Design review of the part built by this model. Coordinates are the model's own, in mm. A direction names the side the tool comes from. Round coordinates to 2 decimals unless told otherwise and drop trailing zeros. Order: outer loops, then holes, each group sorted by start corner. A loop starts at its lowest first (then second) coordinate and runs counter-clockwise, first axis right, second up. Notation, with made-up numbers: (-11.5, 24) - (22.5, 24) arc R28 cw to (22.5, 57) - close; hole circle Ø3 at (1.25, 31). An arc over 180 degrees is marked (long way). Answer as a JSON object with one key per item and string values. Group by question number.
from build123d import *

# Parameters (mm, degrees)
BOSS_EXTRUDE1_DEPTH = 30
SKETCH2_R           = 30
SKETCH2_R_2         = 12.5
CUT_EXTRUDE1_DEPTH  = 146.129146151
BOSS_EXTRUDE2_START = 90
SKETCH3_R           = 12.5
BOSS_EXTRUDE2_DEPTH = 90
BOSS_EXTRUDE3_START = -140
SKETCH3_2_R         = 12.5
BOSS_EXTRUDE3_DEPTH = 90
SKETCH4_W           = 30
SKETCH4_H           = 25
BOSS_EXTRUDE4_DEPTH = 5
SKETCH8_W           = 30
SKETCH8_H           = 5
BOSS_EXTRUDE7_DEPTH = 25
SKETCH9_R           = 4
CUT_EXTRUDE2_DEPTH  = 242.111266906


with BuildPart() as part:
    # Sketch1 → Boss-Extrude1 (new body)
    with BuildSketch(Plane.XY):
        Polygon((20.439052972, 3.783569778), (18.715311494, 3.783569778), (17.077445439, 8.283569778), (15.793733726, 8.283569778), (14.155867672, 3.783569778), (12.432126194, 3.783569778), (10.794260139, 8.283569778), (9.510548426, 8.283569778), (7.872682372, 3.783569778), (6.148940894, 3.783569778), (4.511074839, 8.283569778), (3.227363126, 8.283569778), (1.589497072, 3.783569778), (-0.134244406, 3.783569778), (-1.772110461, 8.283569778), (-3.055822174, 8.283569778), (-4.693688228, 3.783569778), (-6.417429706, 3.783569778), (-8.055295761, 8.283569778), (-9.339007474, 8.283569778), (-10.976873528, 3.783569778), (-12.700615006, 3.783569778), (-14.338481061, 8.283569778), (-15.622192774, 8.283569778), (-17.260058828, 3.783569778), (-18.983800306, 3.783569778), (-20.621666361, 8.283569778), (-21.905378074, 8.283569778), (-23.543244128, 3.783569778), (-25.266985606, 3.783569778), (-26.904851661, 8.283569778), (-28.188563374, 8.283569778), (-29.826429428, 3.783569778), (-31.550170906, 3.783569778), (-33.188036961, 8.283569778), (-34.471748674, 8.283569778), (-36.109614728, 3.783569778), (-37.833356206, 3.783569778), (-39.471222261, 8.283569778), (-40.754933974, 8.283569778), (-42.392800028, 3.783569778), (-44.116541506, 3.783569778), (-45.754407561, 8.283569778), (-47.038119274, 8.283569778), (-48.675985328, 3.783569778), (-50.399726806, 3.783569778), (-52.037592861, 8.283569778), (-53.321304574, 8.283569778), (-54.959170628, 3.783569778), (-56.682912106, 3.783569778), (-58.320778161, 8.283569778), (-59.604489874, 8.283569778), (-61.242355928, 3.783569778), (-62.966097406, 3.783569778), (-64.603963461, 8.283569778), (-65.887675174, 8.283569778), (-67.525541228, 3.783569778), (-69.249282706, 3.783569778), (-70.887148761, 8.283569778), (-72.170860474, 8.283569778), (-73.808726528, 3.783569778), (-75.532468006, 3.783569778), (-77.170334061, 8.283569778), (-78.454045774, 8.283569778), (-80.091911828, 3.783569778), (-81.815653306, 3.783569778), (-83.453519361, 8.283569778), (-84.737231074, 8.283569778), (-86.375097128, 3.783569778), (-88.098838606, 3.783569778), (-89.736704661, 8.283569778), (-91.020416374, 8.283569778), (-92.658282428, 3.783569778), (-94.382023906, 3.783569778), (-96.019889961, 8.283569778), (-97.303601674, 8.283569778), (-98.941467728, 3.783569778), (-100.665209206, 3.783569778), (-102.303075261, 8.283569778), (-103.586786974, 8.283569778), (-105.224653028, 3.783569778), (-106.948394506, 3.783569778), (-108.586260561, 8.283569778), (-109.869972274, 8.283569778), (-111.507838328, 3.783569778), (-113.231579806, 3.783569778), (-114.869445861, 8.283569778), (-116.153157574, 8.283569778), (-117.791023628, 3.783569778), (-118.652894367, 3.783569778), (-118.652894367, -23.716430222), (21.347105633, -23.716430222), (21.347105633, 6.278423959), align=None)
    extrude(amount=BOSS_EXTRUDE1_DEPTH)

    # Sketch2 → Cut-Extrude1 (cut, through all)
    with BuildSketch(Plane.ZY.offset(118.652894367)):
        with Locations((15, -4.216430222)):
            Circle(SKETCH2_R)
        with Locations(Location((15, -4.216430222, 0), (0, 0, 39.7918195))):
            Circle(SKETCH2_R_2, mode=Mode.SUBTRACT)
    extrude(amount=-CUT_EXTRUDE1_DEPTH, mode=Mode.SUBTRACT)

    # Sketch3 → Boss-Extrude2 (add)
    with BuildSketch(Plane.ZY.offset(118.652894367).offset(BOSS_EXTRUDE2_START)):
        with Locations((15, -4.216430222)):
            Circle(SKETCH3_R)
    extrude(amount=-BOSS_EXTRUDE2_DEPTH)

    # Sketch3_2 → Boss-Extrude3 (add)
    with BuildSketch(Plane.ZY.offset(118.652894367).offset(BOSS_EXTRUDE3_START)):
        with Locations((15, -4.216430222)):
            Circle(SKETCH3_2_R)
    extrude(amount=-BOSS_EXTRUDE3_DEPTH)

    # Sketch4 → Boss-Extrude4 (add)
    with BuildSketch(Plane.ZY.offset(208.652894367)):
        with Locations((15, -4.216430222)):
            Rectangle(SKETCH4_W, SKETCH4_H)
    boss_extrude4 = extrude(amount=BOSS_EXTRUDE4_DEPTH)

    # Sketch8 → Boss-Extrude7 (add)
    with BuildSketch(Plane(origin=(0, 8.283569778, 0), x_dir=(1, 0, 0), z_dir=(0, 1, 0))):
        with Locations((-223.652894367, -2.5)):
            Rectangle(SKETCH8_W, SKETCH8_H)
        with Locations((-223.652894367, -27.5)):
            Rectangle(SKETCH8_W, SKETCH8_H)
    boss_extrude7 = extrude(amount=-BOSS_EXTRUDE7_DEPTH)

    # Sketch9 → Cut-Extrude2 (cut, through all)
    with BuildSketch(Plane.XY.offset(30)):
        with Locations((-229.652894367, -4.216430222)):
            Circle(SKETCH9_R)
    cut_extrude2 = extrude(amount=-CUT_EXTRUDE2_DEPTH, mode=Mode.SUBTRACT)

    # Mirror1: Boss-Extrude4, Boss-Extrude7, Cut-Extrude2 across plane
    add(boss_extrude4.mirror(Plane(origin=(-48.652894367, 0, 0), x_dir=(0, 0, 1), z_dir=(1, 0, 0))))
    add(boss_extrude7.mirror(Plane(origin=(-48.652894367, 0, 0), x_dir=(0, 0, 1), z_dir=(1, 0, 0))))
    add(cut_extrude2.mirror(Plane(origin=(-48.652894367, 0, 0), x_dir=(0, 0, 1), z_dir=(1, 0, 0))), mode=Mode.SUBTRACT)


solid = part.part
1. Mouldability with a two-part tool opening along Y and no side actions: class faces 5 (the cylindrical face through (128.532, -3.015, 27.535)), 6 (the flat face through (-224, -4, 0)), 7 (the flat face through (123.2, 8.284, 4.8)) as pulls with the +Y half, pulls with the -Y half, needs draft (parallel to the pull), parting line crosses it, or undercut.
2. Take a section at B-B, the plane x = 101.5. Give the boundary of the cut face in (y, z), then the cut area to 3 significant figures.
3. To check wall thickness, follow line 1 (X direction, y = 0.25, z = 27); line 2 (X direction, y = 0, z = 17.75); line 3 (Y direction, x = -181.5, z = 14.25). State the ranges of each line that lie inside material, in increasing order. Write a range as from..to.
4. Clearance check with flat-ended pins moving along their axes: P1, Ø5, axis at x = -98, y = -11.5, coming from the -Z side; P2, Ø1, axis at y = 0, z = 19, coming from the +X side; P3, Ø8, axis at x = 43, y = -4, coming from the +Z side. State where each tip first meets the part, or that it passes through.
5. Tool access review of faces 1 (the flat face through (126, -4, 25)), 2 (the flat face through (-208.653, -6, 28)), 3 (the flat face through (-208.653, -3, 2)), 4 (the flat face through (-224, -4, 25)): name each direction out of +Z, -Z, +X, -X, +Y, -Y from which nothing blocks a thin tool from reaching the whole face with its end or side.
6. Take a section at A-A, the plane y = -12.5. Give the boundary of the cut face in (x, z), then the cut area to 3 significant figures.
Response values:
{
 "1": {"face 5": "undercut", "face 6": "needs draft", "face 7": "pulls with the +Y half"},
 "2": {"outline": "circle Ø25 at (-4.22, 15)", "area": "491 mm2"},
 "3": {"line 1": "-238.65..-208.65, 111.35..141.35", "line 2": "-213.65..116.35", "line 3": "-16.69..8.26"},
 "4": {"P1": "z = 3.45", "P2": "x = 116.35", "P3": "z = 27.5"},
 "5": {"face 1": "+X, +Y, -Y", "face 2": "+Z", "face 3": "-Z", "face 4": "-X, +Y, -Y"},
 "6": {"outline": "(-238.65, 0) - (-208.65, 0) - (-208.65, 5.64) - (111.35, 5.64) - (111.35, 0) - (141.35, 0) - (141.35, 5) - (116.35, 5) - (116.35, 25) - (141.35, 25) - (141.35, 30) - (111.35, 30) - (111.35, 24.36) - (-208.65, 24.36) - (-208.65, 30) - (-238.65, 30) - (-238.65, 25) - (-213.65, 25) - (-213.65, 5) - (-238.65, 5) - close", "area": "6,790 mm2"}
}
